from build123d import *

# Parameters (mm, degrees)
BOSS_EXTRU_1_DEPTH      = 5
ESQUISSE3_R             = 2.1
ENL_V_MAT_EXTRU_2_DEPTH = 580.22097683


with BuildPart() as part:
    # Esquisse1 → Boss.-Extru.1 (new body)
    with BuildSketch(Plane.XY):
        Polygon((-29.5, 326.885786438), (-29.5, 47.628797826), (21.727899478, 23), (460.5, 23), (460.5, 171.815398059), (422.5, 201.815398059), (422.5, 351.3), (-5.085786438, 351.3), align=None)
    extrude(amount=-BOSS_EXTRU_1_DEPTH)

    # Esquisse3 → Enlèv. mat.-Extru.2 (cut, through all)
    with BuildSketch(Plane.XY):
        with Locations((106.8, 31)):
            Circle(ESQUISSE3_R)
        with Locations((128.8, 31)):
            Circle(ESQUISSE3_R)
        with Locations((372.5, 31)):
            Circle(ESQUISSE3_R)
        with Locations((394.5, 31)):
            Circle(ESQUISSE3_R)
    extrude(amount=-ENL_V_MAT_EXTRU_2_DEPTH, mode=Mode.SUBTRACT)


solid = part.part
Can you work these out from the model? Positions are in its coordinate system, mm. Give positions to 0.01 mm unless a question says otherwise; leave off trailing zeros. Loops run counter-clockwise (first coordinate to the right, second up) from the corner with the lowest first, then second, coordinate; pieces in that order, holes last. Notation, with made-up numbers: (1, -22.5) -> (52, -22.5) arc R29 ccw to (52, 7.5) -> close; hole circle Ø2 at (87.25, 36). An arc over 180 degrees is marked (long way). Return JSON: item names as keys, results as strings.
Q1. I need wall thicknesses on probe 1 along Y at (x, z) = (394.5, -2.1); probe 2 along Y at (x, z) = (373, -4.4); probe 3 along X at (y, z) = (299, -4.45). Which ranges of each line are inside material? Lowest first, please.
Checks:
{"probe 1": "y = 23 to 28.9, 33.1 to 351.3", "probe 2": "y = 23 to 28.96, 33.04 to 351.3", "probe 3": "x = -29.5 to 422.5"}
Q2. I want a section at A-A, the plane z = -2.15. List the corners of the cut face in (x, y) for me.
Checks:
{"outline": "(-29.5, 47.63) -> (21.73, 23) -> (460.5, 23) -> (460.5, 171.82) -> (422.5, 201.82) -> (422.5, 351.3) -> (-5.09, 351.3) -> (-29.5, 326.89) -> close; hole circle Ø4.2 at (106.8, 31); hole circle Ø4.2 at (128.8, 31); hole circle Ø4.2 at (372.5, 31); hole circle Ø4.2 at (394.5, 31)"}
Q3. I want a section at B-B, the plane y = 253. List the corners of the cut face in (x, z) for me.
Checks:
{"outline": "(-29.5, -5) -> (422.5, -5) -> (422.5, 0) -> (-29.5, 0) -> close"}
Q4. For pin 1 Ø2.5 at (x, y) = (106.8, 31) entering from +Z; pin 2 Ø2.5 at (y, z) = (288, -3.5) entering from +X, each with a flat end and sliding along its axis, tell me the tip position at first contact or that it passes through.
Checks:
{"pin 1": "passes through", "pin 2": "stops at x = 422.5"}
Q5. I want a section at C-C, the plane y = 189.5. List the corners of the cut face in (x, z) for me.
Checks:
{"outline": "(-29.5, -5) -> (438.1, -5) -> (438.1, 0) -> (-29.5, 0) -> close"}
